Check sheet for the modelled part. Datum: model origin and axes. Units: mm. Give positions to 0.01 mm unless a question says otherwise; leave off trailing zeros. Order: outer loops, then holes, each group sorted by start corner. A loop starts at its lowest first (then second) coordinate and runs counter-clockwise, first axis right, second up.
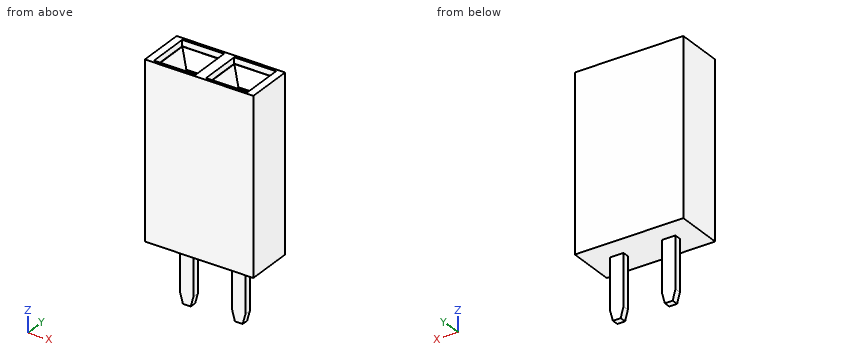
from build123d import *
from OCP.BRepFilletAPI import BRepFilletAPI_MakeChamfer

# Parameters (mm, degrees)
SKETCH_1_W          = 5.3
SKETCH_1_H          = 2.3
EXTRUDE_1_DEPTH     = 4.25
SKETCH_2_W          = 0.8
SKETCH_2_H          = 0.8
CUT_EXTRUDE_1_DEPTH = 8
SKETCH_3_W          = 2.04
SKETCH_3_H          = 2.04
CUT_EXTRUDE_2_DEPTH = 0.3
CHAMFER_1_SIZE      = 0.6
SKETCH_4_W          = 0.65
SKETCH_4_H          = 0.32
EXTRUDE_2_DEPTH     = 3
CHAMFER_2_SIZE      = 0.5
CHAMFER_2_SIZE2     = 0.133974596


with BuildPart() as part:
    # 草图1 → 凸台-拉伸1 (new, symmetric)
    with BuildSketch(Plane.XY):
        Rectangle(SKETCH_1_W, SKETCH_1_H)
    extrude(amount=EXTRUDE_1_DEPTH, both=True)

    # 草图2 → 切除-拉伸1 (cut)
    with BuildSketch(Plane.XY.offset(4.25)):
        with Locations((-1.27, 0)):
            Rectangle(SKETCH_2_W, SKETCH_2_H)
        with Locations((1.27, 0)):
            Rectangle(SKETCH_2_W, SKETCH_2_H)
    extrude(amount=-CUT_EXTRUDE_1_DEPTH, mode=Mode.SUBTRACT)

    # 草图3 → 切除-拉伸2 (cut)
    with BuildSketch(Plane.XY.offset(4.25)):
        with Locations((-1.27, 0)):
            Rectangle(SKETCH_3_W, SKETCH_3_H)
        with Locations((1.27, 0)):
            Rectangle(SKETCH_3_W, SKETCH_3_H)
    extrude(amount=-CUT_EXTRUDE_2_DEPTH, mode=Mode.SUBTRACT)

    # 倒角1
    chamfer_1_edges = [part.edges().sort_by_distance(p)[0] for p in [
        (-1.27, -0.4, 3.95),
        (1.27, -0.4, 3.95),
        (-1.67, 0, 3.95),
        (-1.27, 0.4, 3.95),
        (-0.87, 0, 3.95),
        (1.27, 0.4, 3.95),
        (0.87, 0, 3.95),
        (1.67, 0, 3.95),
    ]]
    chamfer(chamfer_1_edges, length=CHAMFER_1_SIZE)

    # 草图4 → 凸台-拉伸2 (add)
    with BuildSketch(Plane(origin=(0, 0, -4.25), x_dir=(-1, 0, 0), z_dir=(0, 0, -1))):
        with Locations((-1.27, 0)):
            Rectangle(SKETCH_4_W, SKETCH_4_H)
        with Locations((1.27, 0)):
            Rectangle(SKETCH_4_W, SKETCH_4_H)
    extrude(amount=EXTRUDE_2_DEPTH)

    # 倒角2: one chamfer whose edges measure the first distance from different faces: ONE call of the kernel's chamfer builder (chamfer() names one face for all edges)
    chamfer_2_edges_1 = [part.edges().sort_by_distance(p)[0] for p in [
        (1.595, 0, -7.25),
    ]]
    chamfer_2_side_1 = [part.faces().sort_by_distance(p)[0] for p in [
        (1.595, 0, -5.75),
    ]]
    chamfer_2_edges_2 = [part.edges().sort_by_distance(p)[0] for p in [
        (0.945, 0, -7.25),
    ]]
    chamfer_2_side_2 = [part.faces().sort_by_distance(p)[0] for p in [
        (0.945, 0, -5.75),
    ]]
    chamfer_2_edges_3 = [part.edges().sort_by_distance(p)[0] for p in [
        (-0.945, 0, -7.25),
    ]]
    chamfer_2_side_3 = [part.faces().sort_by_distance(p)[0] for p in [
        (-0.945, 0, -5.75),
    ]]
    chamfer_2_edges_4 = [part.edges().sort_by_distance(p)[0] for p in [
        (-1.595, 0, -7.25),
    ]]
    chamfer_2_side_4 = [part.faces().sort_by_distance(p)[0] for p in [
        (-1.595, 0, -5.75),
    ]]
    chamfer_2 = BRepFilletAPI_MakeChamfer(part.part.solid().wrapped)
    for e in chamfer_2_edges_1:
        chamfer_2.Add(CHAMFER_2_SIZE, CHAMFER_2_SIZE2, e.wrapped, chamfer_2_side_1[0].wrapped)  # the first distance lies on this face
    for e in chamfer_2_edges_2:
        chamfer_2.Add(CHAMFER_2_SIZE, CHAMFER_2_SIZE2, e.wrapped, chamfer_2_side_2[0].wrapped)  # the first distance lies on this face
    for e in chamfer_2_edges_3:
        chamfer_2.Add(CHAMFER_2_SIZE, CHAMFER_2_SIZE2, e.wrapped, chamfer_2_side_3[0].wrapped)  # the first distance lies on this face
    for e in chamfer_2_edges_4:
        chamfer_2.Add(CHAMFER_2_SIZE, CHAMFER_2_SIZE2, e.wrapped, chamfer_2_side_4[0].wrapped)  # the first distance lies on this face
    add(Compound.cast(chamfer_2.Shape()), mode=Mode.REPLACE)


solid = part.part
1) Depth check by flat-ended pin: pin 1 Ø0.7 at (x, y) = (0.5, 0) entering from -Z. Enter the tip coordinate at first touch or a pass-through.
Recorded:
pin 1: stops at z = -4.25
2) Section check B-B, the plane z = -1.5. Record the cut outline in (x, y), then the cut area to 3 significant figures.
Recorded:
outline: (-2.65, -1.15) - (2.65, -1.15) - (2.65, 1.15) - (-2.65, 1.15) - close; hole (-1.67, -0.4) - (-0.87, -0.4) - (-0.87, 0.4) - (-1.67, 0.4) - close; hole (0.87, -0.4) - (1.67, -0.4) - (1.67, 0.4) - (0.87, 0.4) - close
area: 10.9 mm2
3) Section check A-A, the plane z = -5.25. Record the cut outline in (x, y) (3 decimals), then the cut area to 3 significant figures.
Recorded:
outline: (-1.595, -0.16) - (-0.945, -0.16) - (-0.945, 0.16) - (-1.595, 0.16) - close; (0.945, -0.16) - (1.595, -0.16) - (1.595, 0.16) - (0.945, 0.16) - close
area: 0.416 mm2
4) Material ranges on L1, parallel to Y at x = -1.6, z = -2.5; L2, parallel to Y at x = 1.25, z = -5.75; L3, parallel to X at y = -0.05, z = -5.75 (3 decimals), recorded low to high.
Recorded:
L1: y = -1.15 to -0.4, 0.4 to 1.15
L2: y = -0.16 to 0.16
L3: x = -1.595 to -0.945, 0.945 to 1.595
